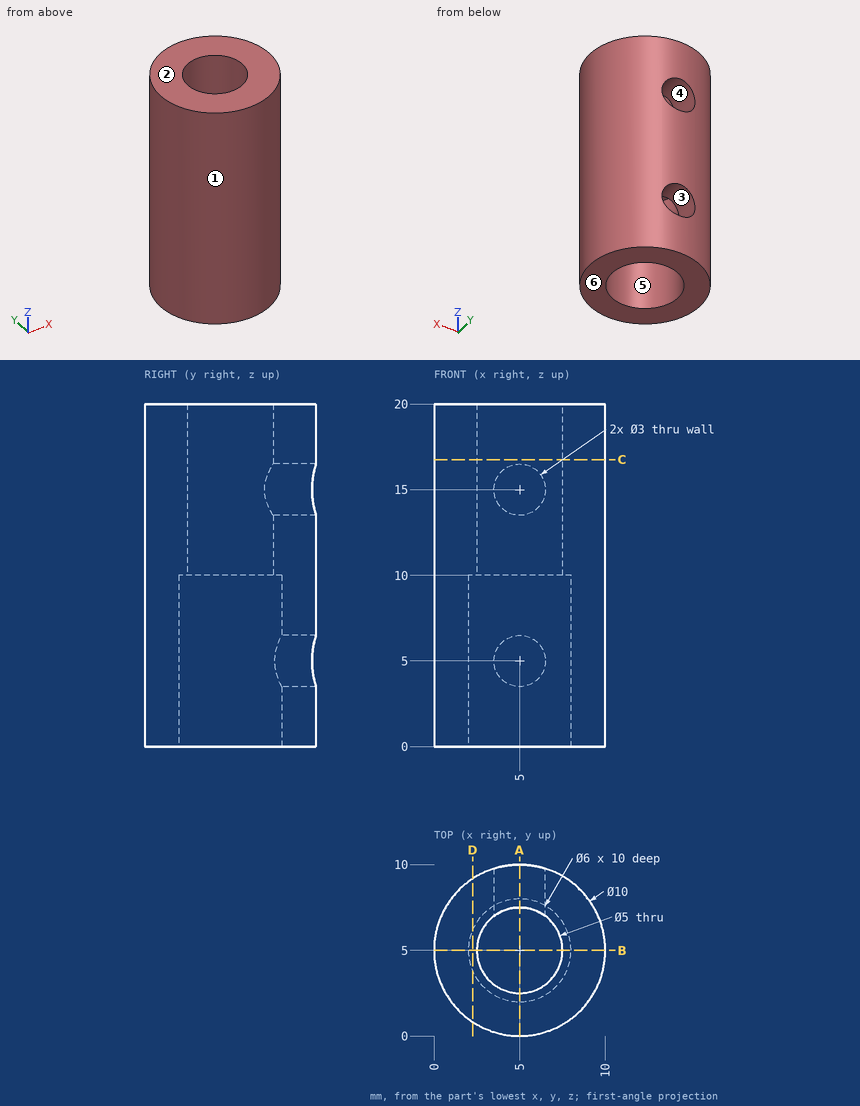
Verification items for this drawing (mm, ordinates from the low corner). A direction names the side the tool comes from. Round coordinates to 2 decimals unless told otherwise and drop trailing zeros. Write each loop counter-clockwise with the first axis right and the second up, starting at its lowest first coordinate (ties: lowest second). Pieces come first, ordered by that corner, then holes. Notation, with made-up numbers: (5.25, 21) - (43.25, 21) arc R33 cw to (43.25, 53) - close; hole circle Ø9 at (87, 35.25). An arc over 180 degrees is marked (long way). Answer as a JSON object with one key per item and string values. Group by question number.
Q1. Section check D-D, the plane x = 2.25. Enter the section's corners in (y, z), plus the area to 3 significant figures.
Q2. Section check C-C, the plane z = 16.75. Enter the section's corners in (x, y).
Q3. Mould release check, pull along X, two halves, no side actions. Record for the marked faces 1, 2 and 3: released by +X, released by -X, zero draft, split by the parting line, or undercut.
Q4. Go/stop test with flat-tipped pins: pin 1 Ø1 at (x, z) = (5.5, 4) entering from -Y; pin 2 Ø1.5 at (x, z) = (1.5, 3.5) entering from +Y; pin 3 Ø3 at (x, z) = (8.5, 6) entering from -Y; pin 4 Ø1.8 at (x, z) = (5, 15) entering from +Y. Record where each tip stops, or that it passes through.
Q5. Tool access check on the marked faces 4, 5 and 6. Record the directions out of +Z, -Z, +X, -X, +Y, -Y that give a thin tool (end or side, any length) a straight path to the whole face; none if there is none.
Q6. Thickness scan on line 1 (Z direction, x = 5, y = 9.25); line 2 (Z direction, x = 4.5, y = 9); line 3 (Y direction, x = 5, z = 17). Record the ranges inside material, lowest first.
Q7. Section check B-B, the plane y = 5. Enter the section's corners in (x, z).
Q8. Section check A-A, the plane x = 5. Enter the section's corners in (y, z).
Found:
{
 "1": {"outline": "(0.82, 0) - (3.8, 0) - (3.8, 10) - (6.2, 10) - (6.2, 0) - (9.18, 0) - (9.18, 20) - (0.82, 20) - close", "area": "143 mm^2"},
 "2": {"outline": "circle Ø10 at (5, 5); hole circle Ø5 at (5, 5)"},
 "3": {"face 1": "split by the parting line", "face 2": "zero draft", "face 3": "undercut"},
 "4": {"pin 1": "stops at y = 0", "pin 2": "stops at y = 9.18", "pin 3": "stops at y = 0.42", "pin 4": "stops at y = 2.67"},
 "5": {"face 4": "+Y", "face 5": "-Z", "face 6": "-Z, +X, -X, +Y, -Y"},
 "6": {"line 1": "z = 0 to 3.5, 6.5 to 13.5, 16.5 to 20", "line 2": "z = 0 to 3.59, 6.41 to 13.59, 16.41 to 20", "line 3": "y = 0 to 2.5, 7.5 to 10"},
 "7": {"outline": "(0, 0) - (2, 0) - (2, 10) - (2.5, 10) - (2.5, 20) - (0, 20) - close; (7.5, 10) - (8, 10) - (8, 0) - (10, 0) - (10, 20) - (7.5, 20) - close"},
 "8": {"outline": "(0, 0) - (2, 0) - (2, 10) - (2.5, 10) - (2.5, 20) - (0, 20) - close; (7.5, 10) - (8, 10) - (8, 6.5) - (10, 6.5) - (10, 13.5) - (7.5, 13.5) - close; (7.5, 16.5) - (10, 16.5) - (10, 20) - (7.5, 20) - close; (8, 0) - (10, 0) - (10, 3.5) - (8, 3.5) - close"}
}
